Here's how the part is built. I have some questions about the finished solid (model axes, mm). Round coordinates to 2 decimals unless told otherwise and drop trailing zeros. Order: outer loops, then holes, each group sorted by start corner. A loop starts at its lowest first (then second) coordinate and runs counter-clockwise, first axis right, second up. Notation, with made-up numbers: M 71.25,53 L 123.25,53 A17 cw 123.25,65 Z; hole C -1,-34.5 d1. An arc over 180 degrees is marked long. Write each question's results on one line, items separated by ' | '. Start each with the question number.
```python
from build123d import *

# Parameters (mm, degrees)
TAPA_R                  = 285
SALIENTE_EXTRUIR1_DEPTH = 6
CROQUIS2_R              = 3.5
CORTAR_EXTRUIR4_DEPTH   = 7


with BuildPart() as part:
    # Tapa → Saliente-Extruir1 (new body)
    with BuildSketch(Plane(origin=(0, 0, 0), x_dir=(1, 0, 0), z_dir=(0, 1, 0))):
        Circle(TAPA_R)
    extrude(amount=SALIENTE_EXTRUIR1_DEPTH)

    # Croquis2 → Cortar-Extruir4 (cut, through all)
    with BuildSketch(Plane(origin=(0, 0, 0), x_dir=(1, 0, 0), z_dir=(0, 1, 0))):
        with Locations((228.035, 0)):
            Circle(CROQUIS2_R)
        with Locations((0, -228.035)):
            Circle(CROQUIS2_R)
        with Locations((-228.035, 0)):
            Circle(CROQUIS2_R)
        with Locations((0, 228.035)):
            Circle(CROQUIS2_R)
    extrude(amount=CORTAR_EXTRUIR4_DEPTH, mode=Mode.SUBTRACT)


solid = part.part
```
(1) I want a section at C-C on z = -139. Write out the boundary of the cut face in (x, y).
(2) I want a section at A-A on y = 2.75. Write out the boundary of the cut face in (x, z) (3 decimals), and give its area (3 significant figures).
(3) I'm going to push flat-ended pins straight in: pin 1 Ø1 at (x, y) = (-42, 5) entering from +Z; pin 2 Ø2 at (x, y) = (129, 5.5) entering from -Z. Where does each tip first touch, or does it pass through?
(4) I want a section at B-B on x = -97.5. Write out the boundary of the cut face in (y, z).
(5) Please list where these lines run through material, in increasing order: line 1 (X direction, y = 2.5, z = 0) (3 decimals); line 2 (Z direction, x = -124.5, y = 3.9).
Solutions:
1) outline: M -248.81,0 L 248.81,0 L 248.81,6 L -248.81,6 Z
2) outline: C 0,0 d570; hole C -228.035,0 d7; hole C 0,-228.035 d7; hole C 0,228.035 d7; hole C 228.035,0 d7 | area: 255,000 mm^2
3) pin 1: z = 281.96 | pin 2: z = -254.64
4) outline: M 0,-267.8 L 6,-267.8 L 6,267.8 L 0,267.8 Z
5) line 1: -285 to -231.535, -224.535 to 224.535, 231.535 to 285 | line 2: -256.37 to 256.37
